Work out the finished part from the listing and answer in its coordinate system (mm). Round coordinates to 2 decimals unless told otherwise and drop trailing zeros. Order: outer loops, then holes, each group sorted by start corner. A loop starts at its lowest first (then second) coordinate and runs counter-clockwise, first axis right, second up. Notation, with made-up numbers: (-18, 19.25) - (25, 19.25) arc R20 ccw to (25, 37.25) - close; hole circle Ø6 at (52.5, -29). An arc over 180 degrees is marked (long way). Use one line per item in the form item = value. Start each with the question number.
Q1. The part is cut by section A-A on x = 0. Determine the outline of the cut face in (y, z), plus the area to 3 significant figures.
Q2. Given P1, Ø2, axis at y = 40.5, z = 10, coming from the -X side; P2, Ø11, axis at x = 2, z = 8, coming from the +Y side; P3, Ø2, axis at x = -3.5, y = -35, coming from the -Z side, each flat-ended and moving along its own axis, determine where each tip first touches the part or whether it passes through.
Q3. The part is cut by section C-C on y = -10. Determine the outline of the cut face in (x, z), plus the area to 3 significant figures.
Q4. Find the intervals of material crossed by line 1 (Z direction, x = -35.5, y = 52); line 2 (Y direction, x = 2, z = 5.5); line 3 (Y direction, x = -56.25, z = 0.85), in increasing order. Write a range as [from, to].
Q5. The part is cut by section B-B on z = 5.5. Determine the outline of the cut face in (x, y), plus the area to 3 significant figures.
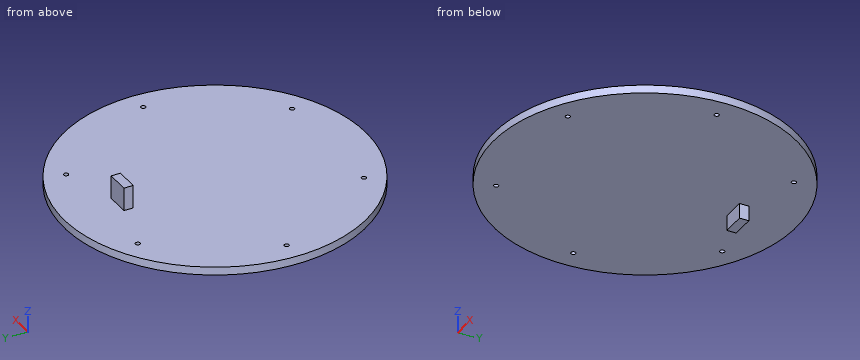
from build123d import *

# Parameters (mm, degrees)
SKETCH_1_R          = 65
EXTRUDE_1_DEPTH     = 3.5
SKETCH_2_W          = 10
SKETCH_2_H          = 4
EXTRUDE_2_DEPTH     = 10
SKETCH_3_R          = 1
CUT_EXTRUDE_1_DEPTH = 10


with BuildPart() as part:
    # 草图1 → 凸台-拉伸1 (new body)
    with BuildSketch(Plane.XY):
        Circle(SKETCH_1_R)
    extrude(amount=EXTRUDE_1_DEPTH)

    # 草图2 → 凸台-拉伸2 (add, symmetric)
    with BuildSketch(Plane.XY.offset(3.5)):
        with Locations((0, 40)):
            Rectangle(SKETCH_2_W, SKETCH_2_H)
    extrude(amount=EXTRUDE_2_DEPTH, both=True)

    # 草图3 → 切除-拉伸1 (cut)
    with BuildSketch(Plane(origin=(0, 0, 0), x_dir=(-1, 0, 0), z_dir=(0, 0, -1))):
        with Locations((56.25, 0)):
            Circle(SKETCH_3_R)
        with Locations((28.125, -48.713928963)):
            Circle(SKETCH_3_R)
        with Locations((-28.125, -48.713928963)):
            Circle(SKETCH_3_R)
        with Locations((-56.25, 0)):
            Circle(SKETCH_3_R)
        with Locations((-28.125, 48.713928963)):
            Circle(SKETCH_3_R)
        with Locations((28.125, 48.713928963)):
            Circle(SKETCH_3_R)
    extrude(amount=-CUT_EXTRUDE_1_DEPTH, mode=Mode.SUBTRACT)


solid = part.part
Found:
q1.outline = (-65, 0) - (38, 0) - (38, -6.5) - (42, -6.5) - (42, 0) - (65, 0) - (65, 3.5) - (42, 3.5) - (42, 13.5) - (38, 13.5) - (38, 3.5) - (-65, 3.5) - close
q1.area = 521 mm²
q2.P1 = -5
q2.P2 = 65
q2.P3 = 0
q3.outline = (-64.23, 0) - (64.23, 0) - (64.23, 3.5) - (-64.23, 3.5) - close
q3.area = 450 mm²
q4.line_1 = [0, 3.5]
q4.line_2 = [38, 42]
q4.line_3 = [-32.57, -1], [1, 32.57]
q5.outline = (-5, 38) - (5, 38) - (5, 42) - (-5, 42) - close
q5.area = 40.0 mm²
